Work out the finished part from the listing and answer in its coordinate system (mm). A direction names the side the tool comes from. Give positions to 0.01 mm unless a question says otherwise; leave off trailing zeros. Loops run counter-clockwise (first coordinate to the right, second up) from the corner with the lowest first, then second, coordinate; pieces in that order, holes last. Notation, with made-up numbers: (31.25, 41) - (58.25, 41) arc R26 ccw to (58.25, 80) - close; hole circle Ø9 at (-4, -8.5). An arc over 180 degrees is marked (long way). One line per question, with ' | ' between items. Start each with the question number.
1. For a pull along Z with two mould halves and no side action, classify faces 1 (the face through (6, 25, -1)), 2 (the face through (2.5, 25.4, -2)), 3 (the face through (2, 25, -3)) as released by +Z, released by -Z, zero draft, split by the parting line, or undercut.
2. Section A-A (x = 0.5) is taken. Determine the outline of the cut face in (y, z).
3. Find the intervals of material crossed by line 1 (X direction, y = 38, z = -0.6); line 2 (Z direction, x = 4.75, y = 20.5), in increasing order.
4. Section B-B (z = -1.1) is taken. Determine the outline of the cut face in (x, y).
5. Which of the six approach directions +Z, -Z, +X, -X, +Y, -Y give full straight-line access (tool end or side, diameter ignored) to faces 4 (the face through (2.5, 25.4, 0)), 5 (the face through (1.7, 51.5, -1))?
6. Section C-C (y = 28) is taken. Determine the outline of the cut face in (x, z), plus the area to 3 significant figures.
from build123d import *

# Parameters (mm, degrees)
SKETCH1_W           = 7
SKETCH1_H           = 4
SKETCH1_W_2         = 1
SKETCH1_H_2         = 2
BOSS_EXTRUDE1_DEPTH = 51.5


with BuildPart() as part:
    # Sketch1 → Boss-Extrude1 (new body)
    with BuildSketch(Plane(origin=(0, 0, 0), x_dir=(1, 0, 0), z_dir=(0, 1, 0))):
        with Locations((2.5, 1)):
            Rectangle(SKETCH1_W, SKETCH1_H)
        with Locations((0.5, 1)):
            Rectangle(SKETCH1_W_2, SKETCH1_H_2, mode=Mode.SUBTRACT)
        with Locations((2.5, 1)):
            Rectangle(SKETCH1_W_2, SKETCH1_H_2, mode=Mode.SUBTRACT)
        with Locations((4.5, 1)):
            Rectangle(SKETCH1_W_2, SKETCH1_H_2, mode=Mode.SUBTRACT)
    extrude(amount=BOSS_EXTRUDE1_DEPTH)


solid = part.part
Conclusion:
1) face 1: zero draft | face 2: undercut | face 3: released by -Z
2) outline: (0, -3) - (51.5, -3) - (51.5, -2) - (0, -2) - close; (0, 0) - (51.5, 0) - (51.5, 1) - (0, 1) - close
3) line 1: -1 to 0, 1 to 2, 3 to 4, 5 to 6 | line 2: -3 to -2, 0 to 1
4) outline: (-1, 0) - (0, 0) - (0, 51.5) - (-1, 51.5) - close; (1, 0) - (2, 0) - (2, 51.5) - (1, 51.5) - close; (3, 0) - (4, 0) - (4, 51.5) - (3, 51.5) - close; (5, 0) - (6, 0) - (6, 51.5) - (5, 51.5) - close
5) face 4: +Y, -Y | face 5: +Z, -Z, +X, -X, +Y
6) outline: (-1, -3) - (6, -3) - (6, 1) - (-1, 1) - close; hole (0, -2) - (1, -2) - (1, 0) - (0, 0) - close; hole (2, -2) - (3, -2) - (3, 0) - (2, 0) - close; hole (4, -2) - (5, -2) - (5, 0) - (4, 0) - close | area: 22.0 mm²
